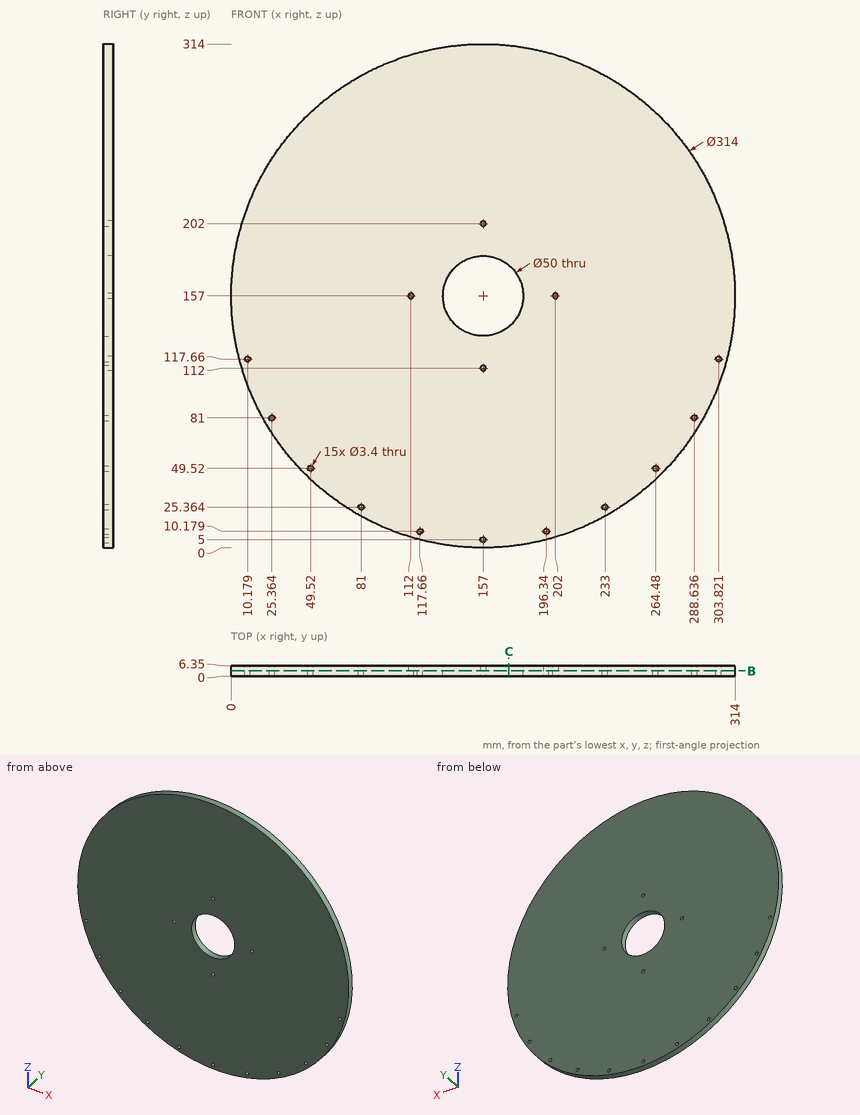
Check sheet for the drawn part. Datum: minimum x, y, z corner. Units: mm. Round coordinates to 2 decimals unless told otherwise and drop trailing zeros. Loops run counter-clockwise (first coordinate to the right, second up) from the corner with the lowest first, then second, coordinate; pieces in that order, holes last. Notation, with made-up numbers: M 34,18.25 L 65,18.25 A27 ccw 65,38.25 Z; hole C 28,75 d11. An arc over 180 degrees is marked long. Write each question's results on one line, items separated by ' | '.
1) Section check B-B on y = 3.25. State how many separate pieces and enclosed holes the cut face has, then the cut area to 3 significant figures.
Checks:
separate pieces: 1 | enclosed holes: 16 | area: 75,300 mm2
2) Gauge pin test, flat ends, axial feed: P1, Ø2.5, axis at x = 117.66, z = 10.18, coming from the +Y side (1 decimal); P2, Ø1.5, axis at x = 137.5, y = 2.5, coming from the -Z side; P3, Ø1.5, axis at x = 198.5, y = 2, coming from the +Z side; P4, Ø1.5, axis at x = 82, y = 3, coming from the +Z side. Record the tip position at first contact, or that the pin passes through.
Checks:
P1: passes through | P2: stops at z = 1.12 | P3: stops at z = 308.62 | P4: stops at z = 295.33
3) Section check C-C on x = 173. Record the boundary of the cut face in (y, z).
Checks:
outline: M 0,0.82 L 6.35,0.82 L 6.35,137.79 L 0,137.79 Z; M 0,176.21 L 6.35,176.21 L 6.35,313.18 L 0,313.18 Z
4) Scan lines: L1, parallel to X at y = 6, z = 49; L2, parallel to X at y = 1, z = 26 (1 decimal); L3, parallel to Z at x = 233, y = 2 (1 decimal). Record each from-to range of solid material in increasing order. Write a range as from..to.
Checks:
L1: x = 43.05..47.9, 51.14..262.86, 266.1..270.95 | L2: x = 70.5..79.4, 82.6..231.4, 234.6..243.5 | L3: z = 19.6..23.7, 27.1..294.4
